from build123d import *

# Parameters (mm, degrees)
PAD_DEPTH    = 4
SKETCH001_R  = 1.5
POCKET_DEPTH = 6
SKETCH004_R  = 1.5
PAD001_DEPTH = 5


with BuildPart() as body001:
    # Sketch003 → Revolution (revolve)
    with BuildSketch(Plane.YZ):
        Polygon((1.6, 5), (4.6, 5), (4.6, -5), (1.6, -5), (4.1, -2.5), (4.1, 2.5), align=None)
    revolve(axis=Axis((0, 0, 0), (0, 0, 1)))


with BuildPart() as cut:
    # Sketch → Pad (new body, symmetric)
    with BuildSketch(Plane.XY):
        Polygon((2.6, 1.501111), (0, 3.002221), (-2.6, 1.501111), (-2.6, -1.501111), (0, -3.002221), (2.6, -1.501111), align=None)
    extrude(amount=PAD_DEPTH, both=True)

    # Sketch001 (on Face8 of Pad) → Pocket (cut)
    with BuildSketch(Plane.XY.offset(4)):
        Circle(SKETCH001_R)
    extrude(amount=-POCKET_DEPTH, mode=Mode.SUBTRACT)

    # Sketch004 (on Face4 of Pocket) → Pad001 (join)
    with BuildSketch(Plane(origin=(0, 0, -4), x_dir=(1, 0, 0), z_dir=(0, 0, -1))):
        Circle(SKETCH004_R)
    extrude(amount=PAD001_DEPTH)

    # Cut: cut Body001
    add(body001.part, mode=Mode.SUBTRACT)


solid = cut.part
Source: CAD feature listing. Evaluate the final solid. Frame: model axes, mm. A direction names the side the tool comes from. Give positions to 0.01 mm unless a question says otherwise; leave off trailing zeros. Write each loop counter-clockwise with the first axis right and the second up, starting at its lowest first coordinate (ties: lowest second). Pieces come first, ordered by that corner, then holes. Notation, with made-up numbers: (30, 53.5) -> (41, 53.5) arc R21 ccw to (41, 82.5) -> close; hole circle Ø3 at (53, -30). An arc over 180 degrees is marked (long way). Return JSON: item names as keys, results as strings. Group by question number.
1. Material intervals for line 1 (Y direction, x = -1.35, z = 2); line 2 (X direction, y = 1, z = -1.5); line 3 (Z direction, x = -0.05, y = -1.25), sorted ascending. Write a range as from..to.
2. Section A-A, the plane z = 0. Output: boundary loops of the cut face in (x, y).
3. Access query for faces 5 (the face through (2, 0, -4)), 6 (the face through (-2.38, -1.36, 3.86)). Directions: +Z, -Z, +X, -X, +Y, -Y. A direction counts if a zero-diameter tool reaches every point of the face in a straight line with its end or side. Return the directions, or none.
4. Section C-C, the plane z = -5.25. Output: boundary loops of the cut face in (x, y).
5. Mould query, pull axis X, two halves, no side actions, for faces 1 (the face through (-2.6, 0, 0)), 2 (the face through (-1.5, 0.07, 1.04)), 3 (the face through (0, 0, -2)), 4 (the face through (1.32, 2.24, 0.06)). Classes: +X half, -X half, draft (parallel to the pull), parting line (faces both ways), or undercut.
6. Pin query (flat end, axial travel): pin 1 Ø1.5 at (y, z) = (-1.5, -4.5) entering from -X; pin 2 Ø3 at (y, z) = (-2.5, -6.5) entering from +X; pin 3 Ø3 at (y, z) = (-2, 0.5) entering from -X; pin 4 Ø1.5 at (x, y) = (0.5, 0.5) entering from +Z. Return the tip coordinate at first contact, or that it passes through.
7. Section B-B, the plane z = -2.5. Output: boundary loops of the cut face in (x, y).
Determined:
{
 "1": {"line 1": "y = -2.22..-0.65, 0.65..2.22", "line 2": "x = -2.6..-1.12, 1.12..2.6", "line 3": "z = -9..-2"},
 "2": {"outline": "(-2.6, -1.5) -> (0, -3) -> (2.6, -1.5) -> (2.6, 1.5) -> (0, 3) -> (-2.6, 1.5) -> close; hole circle Ø3 at (0, 0)"},
 "3": {"face 5": "-Z", "face 6": "+Z, -X, -Y"},
 "4": {"outline": "circle Ø3 at (0, 0)"},
 "5": {"face 1": "-X half", "face 2": "undercut", "face 3": "undercut", "face 4": "+X half"},
 "6": {"pin 1": "stops at x = -2.52", "pin 2": "stops at x = 1.12", "pin 3": "stops at x = -2.6", "pin 4": "stops at z = -2"},
 "7": {"outline": "(-2.6, -1.5) -> (0, -3) -> (2.6, -1.5) -> (2.6, 1.5) -> (0, 3) -> (-2.6, 1.5) -> close"}
}
